Design review of the part shown in the three views and the two pictorial views. Dimensions are in mm from the part's minimum x, y and z. A direction names the side the tool comes from. Give positions to 0.01 mm unless a question says otherwise; leave off trailing zeros. Order: outer loops, then holes, each group sorted by start corner. A loop starts at its lowest first (then second) coordinate and runs counter-clockwise, first axis right, second up. Notation, with made-up numbers: M 0,67.25 L 36,67.25 A23 cw 36,91.25 Z; hole C 50,7.5 d2. An arc over 180 degrees is marked long. Answer as a JSON object with one key per item and string values.
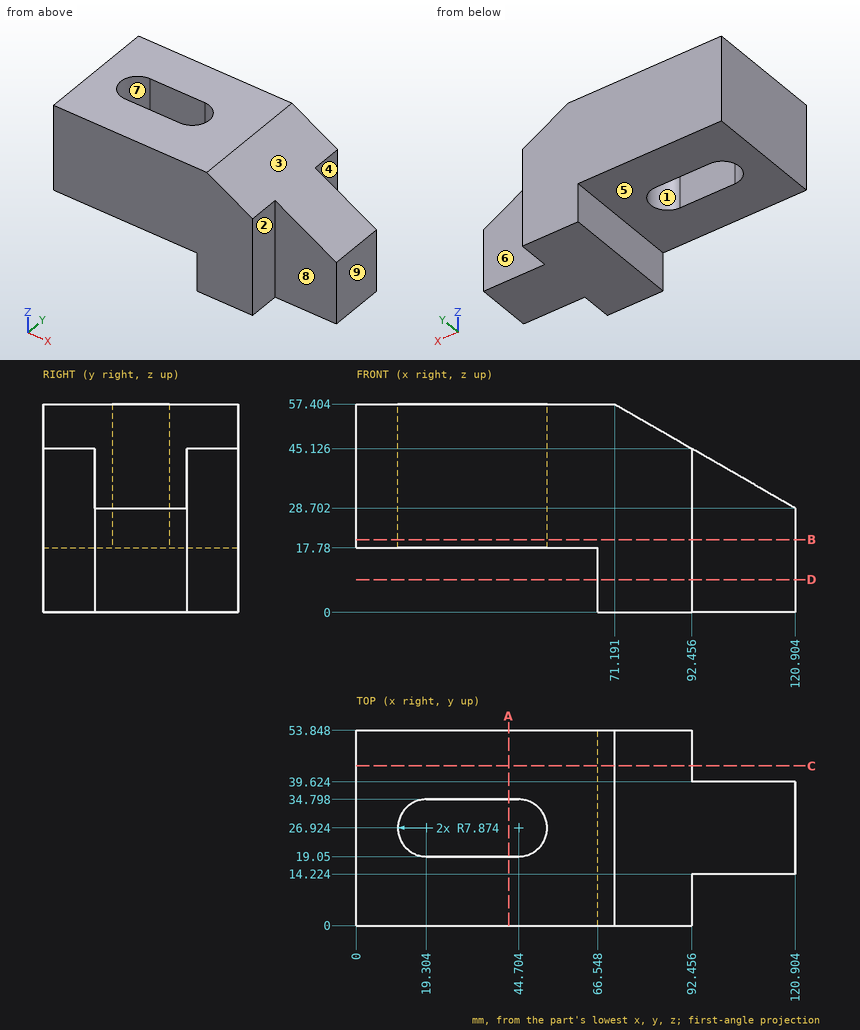
(1) Draft analysis for pull direction Y (two halves, no side actions). For the marked faces 6, 7, 8 and 9, state which applies: +Y half, -Y half, draft (parallel to the pull), parting line (faces both ways), or undercut.
Checked values:
{"face 6": "+Y half", "face 7": "undercut", "face 8": "-Y half", "face 9": "draft"}
(2) We need section D-D (z = 9). Write out the cut boundary in (x, y).
Checked values:
{"outline": "M 66.55,0 L 92.46,0 L 92.46,14.22 L 120.9,14.22 L 120.9,39.62 L 92.46,39.62 L 92.46,53.85 L 66.55,53.85 Z"}
(3) Insertion check: pin 1 (8.5 mm diameter, centred on x = 105, z = 30.5, fed in from +Y); pin 2 (7 mm diameter, centred on y = 46.5, z = 31.5, fed in from +X); pin 3 (5 mm diameter, centred on x = 80, y = 21.5, fed in from +Z). Each pin has a flat end and moves straight along its axis. Give the tip position at first contact, or say it passes through.
Checked values:
{"pin 1": "stops at y = 39.62", "pin 2": "stops at x = 92.46", "pin 3": "stops at z = 53.76"}
(4) We need section A-A (x = 42). Write out the cut boundary in (y, z), plus the area to 3 significant figures.
Checked values:
{"outline": "M 0,17.78 L 19.05,17.78 L 19.05,57.4 L 0,57.4 Z; M 34.8,17.78 L 53.85,17.78 L 53.85,57.4 L 34.8,57.4 Z", "area": "1,510 mm^2"}
(5) To check wall thickness, follow L1, parallel to Y at x = 20.5, z = 20; L2, parallel to X at y = 27.5, z = 27 (1 decimal); L3, parallel to Z at x = 61, y = 46.5. State the ranges of each line that lie inside material, in increasing order. Write a range as from..to.
Checked values:
{"L1": "y = 0..19.05, 34.8..53.85", "L2": "x = 0..11.5, 52.6..120.9", "L3": "z = 17.78..57.4"}
(6) We need section B-B (z = 20). Write out the cut boundary in (x, y), plus the area to 3 significant figures.
Checked values:
{"outline": "M 0,0 L 92.46,0 L 92.46,14.22 L 120.9,14.22 L 120.9,39.62 L 92.46,39.62 L 92.46,53.85 L 0,53.85 Z; hole M 19.3,19.05 L 44.7,19.05 A7.87 ccw 44.7,34.8 L 19.3,34.8 A7.87 ccw Z", "area": "5,110 mm^2"}
(7) Tool access review of the marked faces 1, 2, 3, 4 and 5: name each direction out of +Z, -Z, +X, -X, +Y, -Y from which nothing blocks a thin tool from reaching the whole face with its end or side.
Checked values:
{"face 1": "+Z, -Z", "face 2": "+Z, -Z, +X, -Y", "face 3": "+Z, +X, +Y, -Y", "face 4": "+Z, -Z, +X, +Y", "face 5": "-Z, -X, +Y, -Y"}
(8) We need section C-C (y = 44). Write out the cut boundary in (x, z), plus the area to 3 significant figures.
Checked values:
{"outline": "M 0,17.78 L 66.55,17.78 L 66.55,0 L 92.46,0 L 92.46,45.13 L 71.19,57.4 L 0,57.4 Z", "area": "3,990 mm^2"}
